Build history of the part. All positions in model axes, mm. A direction names the side the tool comes from. Give positions to 0.01 mm unless a question says otherwise; leave off trailing zeros. Loops run counter-clockwise (first coordinate to the right, second up) from the corner with the lowest first, then second, coordinate; pieces in that order, holes last.
1) Two-plate mould, pull along Y, no slides. Class faces 4 (the flat face through (0, 0, -12)), 5 (the cylindrical face through (-0.596, 2.685, 1.359)), 6 (the conical face through (0.065, -0.207, 1.104)): +Y half, -Y half, draft (parallel to the pull), parting line (faces both ways), or undercut.
2) Band-saw the part on A-A on z = -0.5. List the corners of the cut face in (x, y), then the cut area to 3 significant figures.
3) 3-axis set-ups, long thin cutter, end or side, ignore diameter. For faces 1 (the flat face through (1, 2, 0)), 2 (the flat face through (0, 2, 3)), 3 (the flat face through (1.18, 0.7, 2.87)): which of +Z, -Z, +X, -X, +Y, -Y reach the whole face in a straight line?
4) Flat gauge pins, fed straight in: P1, Ø0.7, axis at x = -0.5, y = 1, coming from the +Z side; P2, Ø1, axis at y = 1.5, z = -7, coming from the -X side; P3, Ø0.8, axis at x = -0.5, z = 2, coming from the +Y side. Where does each tip first touch, or does it go through?
5) Wall check: line 1 (X direction, y = 0.1, z = -1.5); line 2 (Z direction, x = 1.75, y = -0.9); line 3 (Y direction, x = -0.35, z = 2.25). Give the ranges that are in metal, low to high.
Autodesk Fusion 360 part; units mm, degrees
sketch "Sketch1" plane through (0, 0, 0) normal (0, 0, 1) x (1, 0, 0)
  circle A0 centre (0, 0) radius 2.75
  line L0 (-0.7217, 1.25) -> (-1.4434, 0)
  line L1 (-1.4434, 0) -> (-0.7217, -1.25)
  line L2 (-0.7217, -1.25) -> (0.7217, -1.25)
  line L3 (0.7217, -1.25) -> (1.4434, 0)
  line L4 (1.4434, 0) -> (0.7217, 1.25)
  line L5 (0.7217, 1.25) -> (-0.7217, 1.25)
  circle A1 centre (0, 0) radius 1.5
  dimension "d5" = 5.5
  dimension "d6" = 1.25
  dimension "d12" = 3
extrude "Extrude1" add sketch "Sketch1" along normal blind 3 contours A0 | L0 L1 L2 L3 L4 L5 | A1
extrude "Extrude2" add sketch "Sketch1" along normal blind 0.75 contours L0 L1 L2 L3 L4 L5
hole "Hole1" at (0, 0, 3) direction (0, 0, -1) diameter 2.5 depth 1.3 tip angle 120
extrude "Extrude3" add sketch "Sketch1" against normal blind 12 contours L0 L1 L2 L3 L4 L5 | A1
extrude "Extrude4" cut sketch "Sketch1" against normal blind 1.3 from surface at 3 contours L0 L1 L2 L3 L4 L5
fillet "Fillet1" radius 0.5 1 edges at (-2.5639, -0.9944, 3)
fillet "Fillet2" radius 0.25 1 edges at (-1.3985, -0.5424, 0)
chamfer "Chamfer1" distance 0.25 angle 45 7 edges at (-1.0825, 0.625, 3) (-1.0825, -0.625, 3) (0, -1.25, 3) (1.0825, -0.625, 3) (1.0825, 0.625, 3) (0, 1.25, 3) (-2.5639, -0.9944, 0)
chamfer "Chamfer2" distance 0.5 angle 45 1 edges at (-1.3985, 0.5424, -12)
thread "Thread1"
equation "Thread_Size = 3 mm"
equation "Thread_Length = 12 mm"
equation "Head_Diameter = 5.5 mm"
equation "Hex_Width = 2.5 mm"
equation "d5 = Head_Diameter"
equation "d6 = Hex_Width / 2"
equation "Head_Height = 3 mm"
equation "d8 = Head_Height"
equation "d10 = Head_Height * 0.25"
equation "d12 = Thread_Size"
equation "d19 = Hex_Depth"
equation "d20 = Hex_Width"
equation "Hex_Depth = 1.3 mm"
properties part number "HW1292SC"
Findings below:
1. face 4: draft
1. face 5: parting line
1. face 6: undercut
2. outline: circle Ø3 at (0, 0)
2. area: 7.07 mm2
3. face 1: -Z
3. face 2: +Z, +X, -X, +Y, -Y
3. face 3: +Z
4. P1: stops at z = 2.85
4. P2: stops at x = -1.12
4. P3: stops at y = 2.75
5. line 1: x = -1.5 to 1.5
5. line 2: z = 0 to 3
5. line 3: y = -2.73 to -1.25, 1.25 to 2.73
